The figure shows three views and two pictorial views of one solid part (mm, origin at its lowest corner). Answer the questions. Coordinates: 2 decimals unless noted, no trailing zeros. Loops run counter-clockwise (first coordinate to the right, second up) from the corner with the lowest first, then second, coordinate; pieces in that order, holes last.
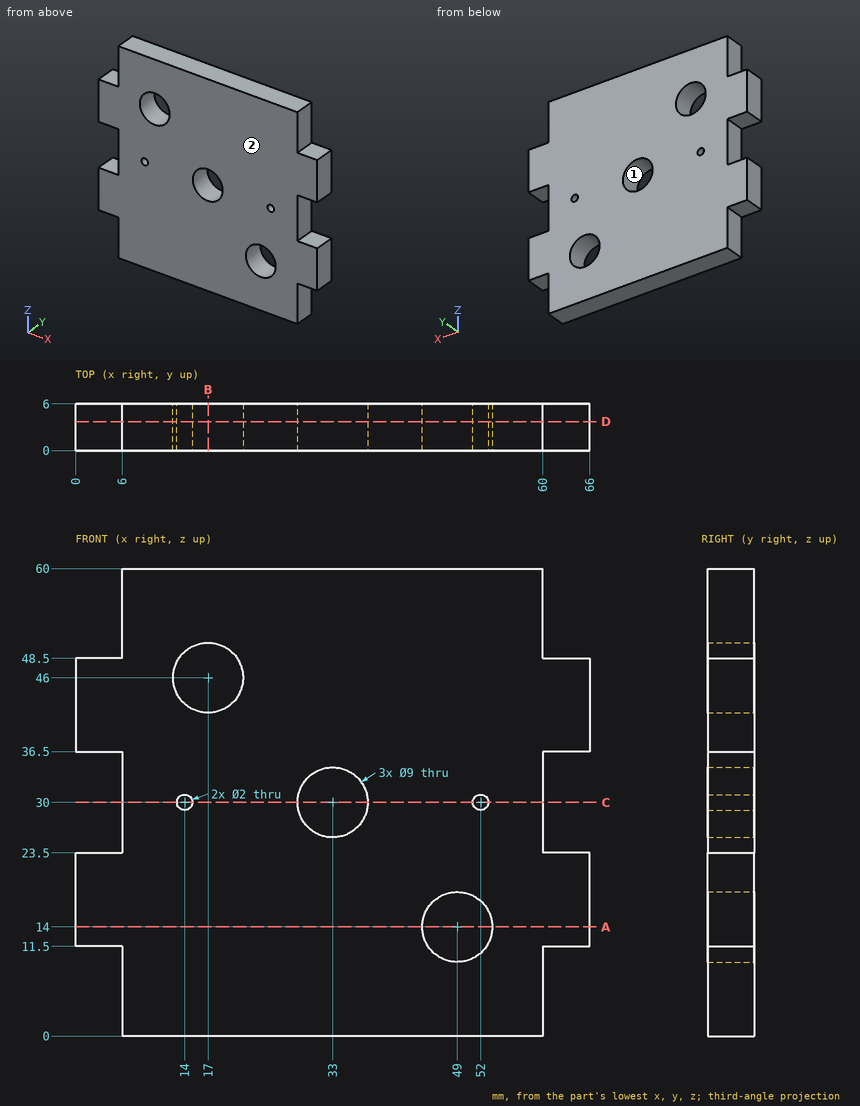
Q1. A cutting plane is placed at D-D (y = 3.75). Give the vertices of the cut face in (x, z), then the cut area to 3 significant figures.
Findings below:
outline: (0, 11.5) - (6, 11.5) - (6, 0) - (60, 0) - (60, 11.5) - (66, 11.5) - (66, 23.5) - (60, 23.5) - (60, 36.5) - (66, 36.5) - (66, 48.5) - (60, 48.5) - (60, 60) - (6, 60) - (6, 48.5) - (0, 48.5) - (0, 36.5) - (6, 36.5) - (6, 23.5) - (0, 23.5) - close; hole circle Ø9 at (17, 46); hole circle Ø2 at (14, 30); hole circle Ø9 at (33, 30); hole circle Ø9 at (49, 14); hole circle Ø2 at (52, 30)
area: 3,330 mm2
Q2. A cutting plane is placed at C-C (z = 30). Give the vertices of the cut face in (x, y).
Findings below:
outline: (6, 0) - (13, 0) - (13, 6) - (6, 6) - close; (15, 0) - (28.5, 0) - (28.5, 6) - (15, 6) - close; (37.5, 0) - (51, 0) - (51, 6) - (37.5, 6) - close; (53, 0) - (60, 0) - (60, 6) - (53, 6) - close
Q3. Straight lines are drawn through the part: probe 1 along X at (y, z) = (4.5, 30); probe 2 along X at (y, z) = (2.9, 46); probe 3 along Z at (x, y) = (33, 4.7). For each, find the intervals that lie inside material, in ascending order.
Findings below:
probe 1: x = 6 to 13, 15 to 28.5, 37.5 to 51, 53 to 60
probe 2: x = 0 to 12.5, 21.5 to 66
probe 3: z = 0 to 25.5, 34.5 to 60
Q4. Flat-ended cylindrical pins translate along their axes: pin 1 Ø1.8 at (x, y) = (2, 1.5) entering from -Z; pin 2 Ø11.5 at (x, z) = (17, 46) entering from +Y; pin 3 Ø1.8 at (y, z) = (2.5, 4.5) entering from +X; pin 4 Ø3 at (y, z) = (3.5, 5.5) entering from -X. Find the tip coordinate at first contact, or state that the pin passes through.
Findings below:
pin 1: stops at z = 11.5
pin 2: stops at y = 6
pin 3: stops at x = 60
pin 4: stops at x = 6
Q5. A cutting plane is placed at A-A (z = 14). Give the vertices of the cut face in (x, y).
Findings below:
outline: (0, 0) - (44.5, 0) - (44.5, 6) - (0, 6) - close; (53.5, 0) - (66, 0) - (66, 6) - (53.5, 6) - close
Q6. A cutting plane is placed at B-B (x = 17). Give the vertices of the cut face in (y, z).
Findings below:
outline: (0, 0) - (6, 0) - (6, 41.5) - (0, 41.5) - close; (0, 50.5) - (6, 50.5) - (6, 60) - (0, 60) - close
Q7. Determine the mould class of the marked faces 1 and 2 for opening direction X: +X half, -X half, draft (parallel to the pull), parting line (faces both ways), or undercut.
Findings below:
face 1: undercut
face 2: draft
